The drawing under review shows one solid part. Ordinate dimensions are in mm from its lowest x, y, z. A direction names the side the tool comes from. Round coordinates to 2 decimals unless told otherwise and drop trailing zeros. Order: outer loops, then holes, each group sorted by start corner. A loop starts at its lowest first (then second) coordinate and runs counter-clockwise, first axis right, second up.
1) Consider section D-D (y = 10.5). Give the boundary of the cut face in (x, z), then the cut area to 3 significant figures.
2) Mouldability with a two-part tool opening along X and no side actions: class the marked faces 4, 5, 6 and 7 as pulls with the +X half, pulls with the -X half, needs draft (parallel to the pull), parting line crosses it, or undercut.
3) To check wall thickness, follow L1, parallel to Z at x = 48, y = 20; L2, parallel to Z at x = 52.95, y = 20; L3, parallel to Z at x = 15, y = 20. State the ranges of each line that lie inside material, in increasing order.
4) Clearance check with flat-ended pins moving along their axes: P1, Ø9, axis at y = 20, z = 40.1, coming from the -X side; P2, Ø7.5, axis at x = 32, y = 15.5, coming from the -Z side; P3, Ø1.8, axis at y = 19.5, z = 33.5, coming from the -X side; P4, Ø19, axis at y = 20, z = 15, coming from the -X side. State where each tip first meets the part, or that it passes through.
5) Consider section A-A (z = 15). Give the boundary of the cut face in (x, y), then the cut area to 3 significant figures.
6) Machinability: for the marked faces 1, 2 and 3, which of the approach directions +Z, -Z, +X, -X, +Y, -Y give a long, thin tool a straight path to every point of the face, cutting with its end or side? Answer none if there is none.
7) Consider section B-B (x = 9). Give the boundary of the cut face in (y, z), then the cut area to 3 significant figures.
8) Consider section C-C (y = 20). Give the number of separate pieces and of enclosed holes in the cut face, then the cut area to 3 significant figures.
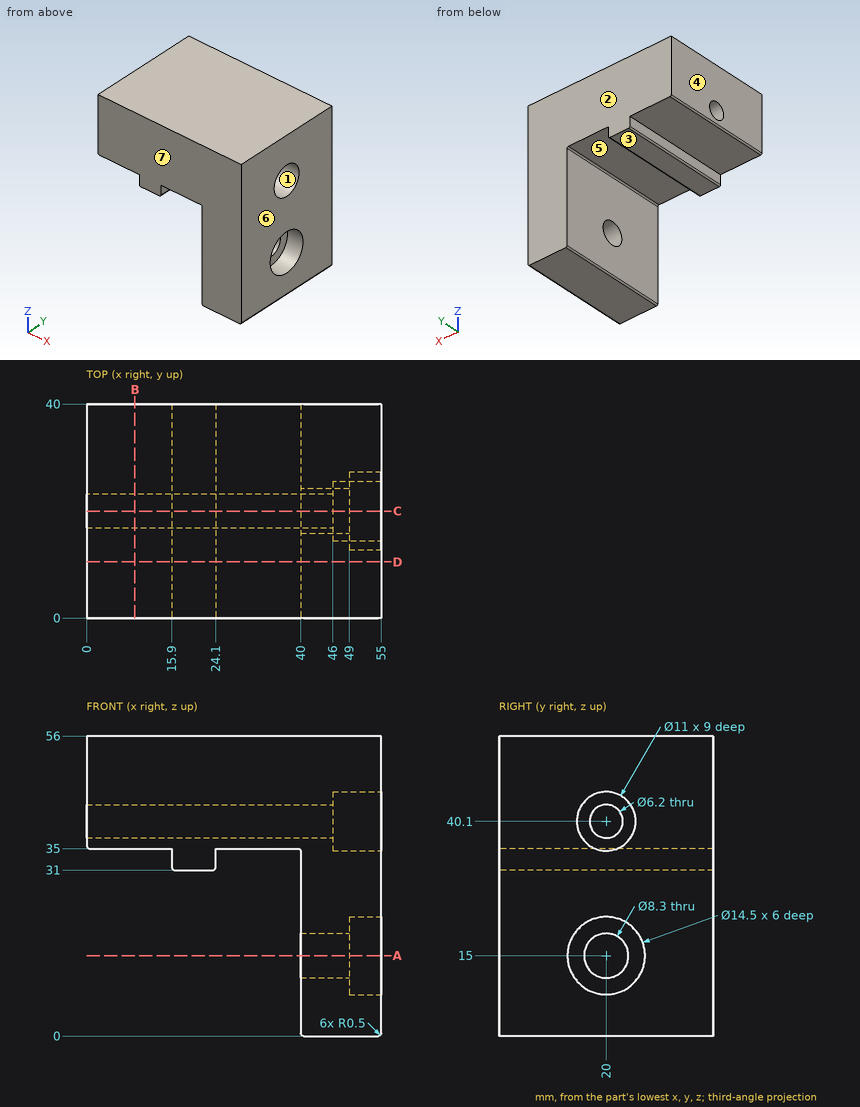
Answer below:
1. outline: (0, 35.5) arc R0.5 ccw to (0.5, 35) - (15.9, 35) - (15.9, 31.5) arc R0.5 ccw to (16.4, 31) - (23.6, 31) arc R0.5 ccw to (24.1, 31.5) - (24.1, 35) - (39.5, 35) arc R0.5 cw to (40, 34.5) - (40, 0.5) arc R0.5 ccw to (40.5, 0) - (54.5, 0) arc R0.5 ccw to (55, 0.5) - (55, 56) - (0, 56) - close
1. area: 1,710 mm2
2. face 4: pulls with the -X half
2. face 5: undercut
2. face 6: pulls with the +X half
2. face 7: needs draft
3. L1: z = 0 to 10.85, 19.15 to 34.6, 45.6 to 56
3. L2: z = 0 to 7.75, 22.25 to 34.6, 45.6 to 56
3. L3: z = 35 to 37, 43.2 to 56
4. P1: stops at x = 0
4. P2: stops at z = 35
4. P3: stops at x = 15.9
4. P4: stops at x = 40
5. outline: (40, 0) - (55, 0) - (55, 12.75) - (49, 12.75) - (49, 15.85) - (40, 15.85) - close; (40, 24.15) - (49, 24.15) - (49, 27.25) - (55, 27.25) - (55, 40) - (40, 40) - close
5. area: 438 mm2
6. face 1: +X
6. face 2: +Z, -Z, +X, -X, +Y
6. face 3: -Z, -X, +Y, -Y
7. outline: (0, 35) - (40, 35) - (40, 56) - (0, 56) - close; hole circle Ø6.2 at (20, 40.1)
7. area: 810 mm2
8. separate pieces: 3
8. enclosed holes: 0
8. area: 1,170 mm2
